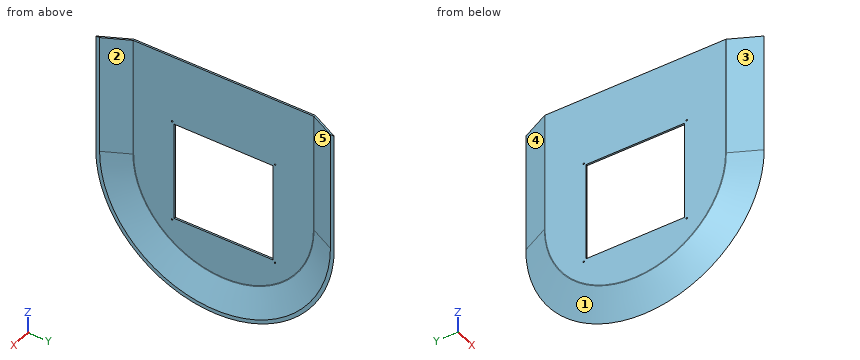
from build123d import *

# Parameters (mm, degrees)
REVOLVE1_ANGLE           = 180
BOSS_EXTRUDE1_DEPTH      = 350
SHELL2_T                 = -5
SKETCH4_W                = 290
SKETCH4_H                = 290
CUT_EXTRUDE1_DEPTH       = 497.747272869
M4_CLEARANCE_HOLE1_D     = 4.5
M4_CLEARANCE_HOLE1_DEPTH = 30
M4_CLEARANCE_HOLE1_TIP   = 1.351936393
FILLET1_R                = 5


with BuildPart() as part:
    # Esquisse2 → Revolve1 (revolve)
    with BuildSketch(Plane.XY):
        Polygon((41.926758797, 350), (41.926758797, 0), (0, 0), (0, 266.190547052), align=None)
    revolve(axis=Axis((41.926758797, 0, 0), (-1, 0, 0)), revolution_arc=REVOLVE1_ANGLE)

    # Sketch5 → Boss-Extrude1 (add)
    with BuildSketch(Plane.XY):
        Polygon((0, 266.190547052), (41.926758797, 350), (41.926758797, -350), (0, -266.190547052), align=None)
    extrude(amount=BOSS_EXTRUDE1_DEPTH)

    # Shell2
    shell2_openings = [part.faces().sort_by_distance(p)[0] for p in [
        (21.913804754, 0, 350),
        (41.926758797, 0, 32.672450622),
    ]]
    offset(amount=SHELL2_T, openings=shell2_openings, kind=Kind.INTERSECTION)

    # Sketch4 → Cut-Extrude1 (cut, through all)
    with BuildSketch(Plane.ZY):
        Rectangle(SKETCH4_W, SKETCH4_H)
    extrude(amount=-CUT_EXTRUDE1_DEPTH, mode=Mode.SUBTRACT)

    # M4 Clearance Hole1
    with Locations(Plane.ZY):
        with Locations((151, 151), (151, -151), (-151, -151), (-151, 151)):
            Hole(M4_CLEARANCE_HOLE1_D / 2, depth=M4_CLEARANCE_HOLE1_DEPTH)
            with Locations((0, 0, -(M4_CLEARANCE_HOLE1_DEPTH + M4_CLEARANCE_HOLE1_TIP / 2))):  # 118° drill point
                Cone(0, M4_CLEARANCE_HOLE1_D / 2, M4_CLEARANCE_HOLE1_TIP, mode=Mode.SUBTRACT)

    # Fillet1
    fillet1_edges = [part.edges().sort_by_distance(p)[0] for p in [
        (0, 266.190547052, 175),
        (0, -266.190547052, 175),
        (5, 0, -265.009652137),
        (5, 265.009652137, 175),
        (5, -265.009652137, 175),
        (0, 0, -266.190547052),
    ]]
    fillet(fillet1_edges, radius=FILLET1_R)


solid = part.part
Design review of the part built by this model. Coordinates are the model's own, in mm. Face numbers are marked on the shaded views. A direction names the side the tool comes from. Coordinates: 2 decimals unless noted, no trailing zeros. Order: outer loops, then holes, each group sorted by start corner. A loop starts at its lowest first (then second) coordinate and runs counter-clockwise, first axis right, second up.
Item 1: The part is to be moulded in two halves that separate along Y. For the marked faces 3, 4 and 5, say which applies: pulls with the +Y half, pulls with the -Y half, needs draft (parallel to the pull), parting line crosses it, or undercut.
Item 2: For the marked faces 1 and 2, list the 3-axis set-ups (+Z, -Z, +X, -X, +Y, -Y) from which the entire face can be reached by the end or side of a thin tool; tool diameter is ignored.
Item 3: Take a section at D-D, the plane x = 23.5. Write out the cut boundary in (y, z).
Item 4: Take a section at B-B, the plane z = 244.5. Write out the cut boundary in (x, y), then the cut area to 3 significant figures.
Item 5: Take a section at A-A, the plane y = 0. Write out the cut boundary in (x, z).
Item 6: For pin 1 Ø10 at (x, z) = (31, 93.5) entering from -Y; pin 2 Ø1 at (y, z) = (24.5, -276.5) entering from -X; pin 3 Ø1.5 at (x, z) = (3, -39.5) entering from +Y; pin 4 Ø4 at (y, z) = (-151, 151) entering from -X, all flat-tipped, find the tip position at first contact; note any pin that passes through.
Item 7: Take a section at C-C, the plane z = 69.5. Write out the cut boundary in (x, y).
Item 8: For line 1 (Y direction, x = 1.35, z = -151); line 2 (Z direction, x = 1.4, y = 151); line 3 (Y direction, x = 3, z = 151), list the stretches that pass through material, from the lowest coordinate up.
The answers:
1. face 3: pulls with the -Y half
1. face 4: pulls with the +Y half
1. face 5: undercut
2. face 1: -Z, -X
2. face 2: +Z, +X
3. outline: (-313.17, 0) arc R313.17 ccw to (313.17, 0) - (313.17, 350) - (301.99, 350) - (301.99, 0) arc R301.99 cw to (-301.99, 0) - (-301.99, 350) - (-313.17, 350) - close
4. outline: (0, -265.01) arc R5 ccw to (0.53, -267.25) - (41.93, -350) - (41.93, -338.82) - (5.53, -266.07) arc R5 cw to (5, -263.83) - (5, 263.83) arc R5 cw to (5.53, 266.07) - (41.93, 338.82) - (41.93, 350) - (0.53, 267.25) arc R5 ccw to (0, 265.01) - close
4. area: 3,540 mm2
5. outline: (0, -265.01) arc R5 ccw to (0.53, -267.25) - (41.93, -350) - (41.93, -338.82) - (5.53, -266.07) arc R5 cw to (5, -263.83) - (5, -145) - (0, -145) - close; (0, 145) - (5, 145) - (5, 350) - (0, 350) - close
6. pin 1: stops at y = -338.15
6. pin 2: stops at x = 5.45
6. pin 3: stops at y = 270.83
6. pin 4: passes through
7. outline: (0, -265.01) arc R5 ccw to (0.53, -267.25) - (41.93, -350) - (41.93, -338.82) - (5.53, -266.07) arc R5 cw to (5, -263.83) - (5, -145) - (0, -145) - close; (0, 145) - (5, 145) - (5, 263.83) arc R5 cw to (5.53, 266.07) - (41.93, 338.82) - (41.93, 350) - (0.53, 267.25) arc R5 ccw to (0, 265.01) - close
8. line 1: y = -222.49 to -153.25, -148.75 to 148.75, 153.25 to 222.49
8. line 2: z = -222.61 to -153.25, -148.75 to 148.75, 153.25 to 350
8. line 3: y = -272.19 to -153.25, -148.75 to 148.75, 153.25 to 272.19
